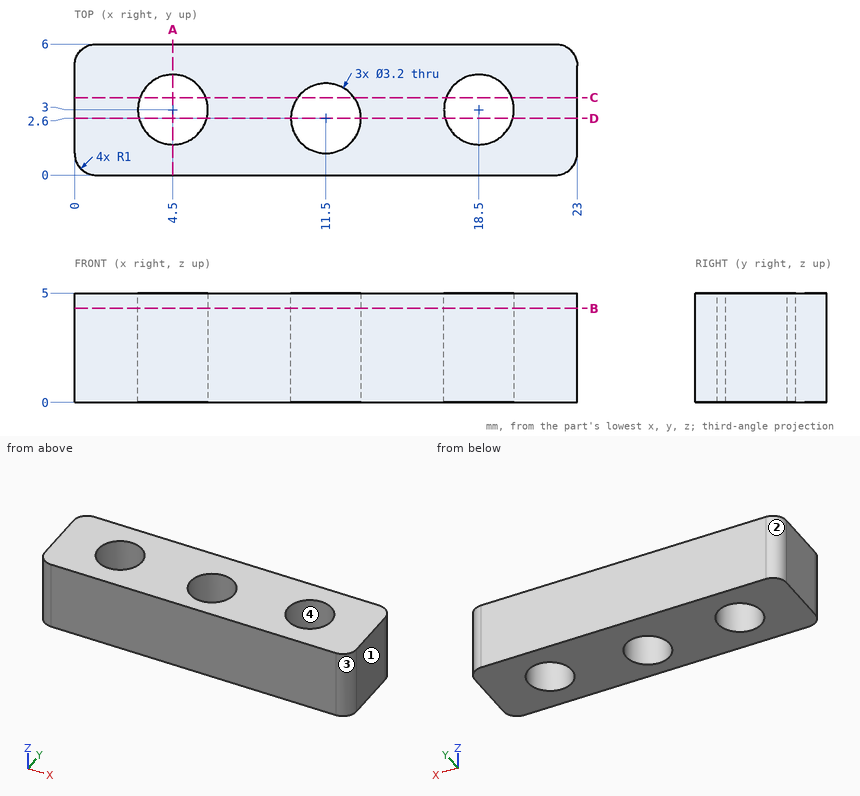
Geometry check sheet. Reference: drawing and pictorial views, mm from the part's lowest x, y, z. Give positions to 0.01 mm unless a question says otherwise; leave off trailing zeros. Order: outer loops, then holes, each group sorted by start corner. A loop starts at its lowest first (then second) coordinate and runs counter-clockwise, first axis right, second up. Notation, with made-up numbers: M 18.25,81.5 L 75.25,81.5 A16 ccw 75.25,95.5 Z; hole C 6.5,28 d11. An arc over 180 degrees is marked long. Answer as a JSON object with one key per item and string values. Group by question number.
1) Cross-section at B-B (z = 4.3). Enter the section's corners in (x, y), then the cut area to 3 significant figures.
2) Scan lines: line 1 along Y through (x, z) = (11.5, 1.15); line 2 along X through (y, z) = (2.7, 2.8); line 3 along X through (y, z) = (1.85, 0.75). Record each from-to range of solid material in increasing order. Write a range as [from, to].
3) Cross-section at D-D (y = 2.6). Enter the section's corners in (x, z).
4) Mould release check, pull along Y, two halves, no side actions. Record for the marked faces 1, 2, 3 and 4: released by +Y, released by -Y, zero draft, split by the parting line, or undercut.
5) Cross-section at A-A (x = 4.5). Enter the section's corners in (y, z), then the cut area to 3 significant figures.
6) Cross-section at C-C (y = 3.55). Enter the section's corners in (x, z).
Result sheet:
{
 "1": {"outline": "M 0,1 A1 ccw 1,0 L 22,0 A1 ccw 23,1 L 23,5 A1 ccw 22,6 L 1,6 A1 ccw 0,5 Z; hole C 4.5,3 d3.2; hole C 11.5,2.6 d3.2; hole C 18.5,3 d3.2", "area": "113 mm2"},
 "2": {"line 1": "y = [0, 1], [4.2, 6]", "line 2": "x = [0, 2.93], [6.07, 9.9], [13.1, 16.93], [20.07, 23]", "line 3": "x = [0, 3.39], [5.61, 10.09], [12.91, 17.39], [19.61, 23]"},
 "3": {"outline": "M 0,0 L 2.95,0 L 2.95,5 L 0,5 Z; M 6.05,0 L 9.9,0 L 9.9,5 L 6.05,5 Z; M 13.1,0 L 16.95,0 L 16.95,5 L 13.1,5 Z; M 20.05,0 L 23,0 L 23,5 L 20.05,5 Z"},
 "4": {"face 1": "zero draft", "face 2": "released by +Y", "face 3": "released by -Y", "face 4": "undercut"},
 "5": {"outline": "M 0,0 L 1.4,0 L 1.4,5 L 0,5 Z; M 4.6,0 L 6,0 L 6,5 L 4.6,5 Z", "area": "14.0 mm2"},
 "6": {"outline": "M 0,0 L 3,0 L 3,5 L 0,5 Z; M 6,0 L 10.21,0 L 10.21,5 L 6,5 Z; M 12.79,0 L 17,0 L 17,5 L 12.79,5 Z; M 20,0 L 23,0 L 23,5 L 20,5 Z"}
}
